Build history of the part. All positions in model axes, mm. A direction names the side the tool comes from. Coordinates: 2 decimals unless noted, no trailing zeros. Loops run counter-clockwise (first coordinate to the right, second up) from the corner with the lowest first, then second, coordinate; pieces in that order, holes last.
(1) Tool access for faces 1 (the face through (-151.49, 51.39, 24.45)), 2 (the face through (-77.27, 0.91, 24.45)), 3 (the face through (-75, 98.425, 5)), 4 (the face through (-75, 6.35, 19)), 5 (the face through (-0.91, 51.39, 24.45)): list every direction of +Z, -Z, +X, -X, +Y, -Y with a clear straight run to the whole face (end or side of a thin tool).
(2) Flat gauge pins, fed straight in: P1, Ø2.5, axis at x = -66.5, y = 5, coming from the +Z side; P2, Ø23, axis at x = -71.5, y = 43, coming from the -Z side (3 decimals); P3, Ø0.8, axis at x = -13.5, z = 26.5, coming from the +Y side. Where does each tip first touch, or does it go through?
(3) Slice it at B-B (x = -34.5). Give the cut face in (y, z) (3 decimals), and give its area (3 significant figures).
(4) Slice it at A-A (z = 4). Give the cut face in (x, y) (3 decimals), and give its area (3 significant figures).
(5) Wall check: L1, parallel to Y at x = -60, z = 16 (3 decimals); L2, parallel to X at y = 44, z = 14 (3 decimals); L3, parallel to X at y = 55.5, z = 26.75. Give the ranges that are in metal, low to high.
(6) Two-plate mould, pull along Y, no slides. Class faces 6 (the face through (-75, 5, 25.4)), 7 (the face through (-77.27, 100.69, 24.45)), 8 (the face through (-77, 94, 9.525)): pulls with the +Y half, pulls with the -Y half, needs draft (parallel to the pull), parting line crosses it, or undercut.
(7) Slice it at C-C (y = 21). Give the cut face in (x, z) (3 decimals).
from build123d import *

# Parameters (mm, degrees)
F0_W        = 101.6
F0_H        = 25.4
F1_DEPTH    = 152.4
F2_W        = 2.54
F2_H        = 12.7
F3_DEPTH    = 152.401
F4_W        = 1.524
F4_H        = 71.12
F5_DEPTH    = 2.54
F6_R        = 3.175
F7_T        = 3.175
F7_T3_DEPTH = 158.75
F7_T5_DEPTH = 77.47
F7_T7_DEPTH = 7.874
F7_T9_DEPTH = 7.874


# Not quite as in the source:
# - a shell that OpenCascade refuses in one call is made with other operations: the cavity is built on its own and cut out


with BuildPart() as f1:
    # F0 (on Right) → F1 (new body)
    with BuildSketch(Plane.YZ):
        with Locations((50.8, 12.7)):
            Rectangle(F0_W, F0_H)
    extrude(amount=-F1_DEPTH)

    # F2 (on face) → F3 (cut, through all)
    with BuildSketch(Plane.YZ):
        with Locations((7.62, 19.05)):
            Rectangle(F2_W, F2_H)
        with Locations((93.98, 19.05)):
            Rectangle(F2_W, F2_H)
    extrude(amount=-F3_DEPTH, mode=Mode.SUBTRACT)

    # F4 (on face) → F5 (join)
    with BuildSketch(Plane.XY.offset(25.4)):
        with Locations((-138.938, 50.8)):
            Rectangle(F4_W, F4_H)
        with Locations((-13.462, 50.8)):
            Rectangle(F4_W, F4_H)
    extrude(amount=F5_DEPTH)

    # F6
    f6_edges = [f1.edges().sort_by_distance(p)[0] for p in [
        (-76.2, 0, 25.4),
        (-76.2, 101.6, 25.4),
        (0, 50.8, 25.4),
        (-152.4, 50.8, 25.4),
    ]]
    fillet(f6_edges, radius=F6_R)

    # F7: shell of thickness 3.175, made by hand


with BuildPart() as f7_core1:
    # F7_t2: copy of F1
    add(f1.part)

    # the walls: a layer under each face that stays
    f7_faces = [f7_core1.faces().sort_by_distance(p)[0] for p in [
        (-76.2, 0, 11.1125),
        (0, 50.8, 12.7),
        (-152.4, 50.8, 12.7),
        (-76.2, 4.7625, 25.4),
        (-76.2, 6.35, 19.05),
        (-76.2, 7.62, 12.7),
        (-76.2, 8.89, 19.05),
        (-76.2, 101.6, 11.1125),
        (-76.2, 92.71, 19.05),
        (-76.2, 96.8375, 25.4),
        (-76.2, 93.98, 12.7),
        (-76.2, 95.25, 19.05),
        (-76.2, 50.8, 25.4),
        (-138.176, 50.8, 26.67),
        (-138.938, 86.36, 26.67),
        (-139.7, 50.8, 26.67),
        (-138.938, 15.24, 26.67),
        (-12.7, 50.8, 26.67),
        (-13.462, 86.36, 26.67),
        (-14.224, 50.8, 26.67),
        (-13.462, 15.24, 26.67),
        (-138.938, 50.8, 27.94),
        (-13.462, 50.8, 27.94),
    ]]
    thicken(f7_faces, amount=-F7_T, mode=Mode.SUBTRACT)

    # F7_s4 → F7_t3 (cut)
    with BuildSketch(Plane.YZ.offset(-155.575)):
        Polygon((6.38175, 12.73175), (3.175, 12.7), (3.175, 9.525), (6.35, 9.525), align=None)
        Polygon((8.85825, 12.73175), (8.89, 9.525), (12.065, 9.525), (12.065, 12.7), align=None)
        Polygon((92.74175, 12.73175), (89.535, 12.7), (89.535, 9.525), (92.71, 9.525), align=None)
        Polygon((95.21825, 12.73175), (95.25, 9.525), (98.425, 9.525), (98.425, 12.7), align=None)
    extrude(amount=F7_T3_DEPTH, mode=Mode.SUBTRACT)

    # F7_s6 → F7_t5 (cut)
    with BuildSketch(Plane.XZ.offset(-89.535)):
        Polygon((-138.14425, 25.43175), (-138.176, 22.225), (-141.351, 22.225), (-141.351, 25.4), align=None)
        Polygon((-139.73175, 25.43175), (-139.7, 22.225), (-136.525, 22.225), (-136.525, 25.4), align=None)
        Polygon((-12.66825, 25.43175), (-12.7, 22.225), (-15.875, 22.225), (-15.875, 25.4), align=None)
        Polygon((-14.25575, 25.43175), (-14.224, 22.225), (-11.049, 22.225), (-11.049, 25.4), align=None)
    extrude(amount=F7_T5_DEPTH, mode=Mode.SUBTRACT)

    # F7_s8 → F7_t7 (cut)
    with BuildSketch(Plane.YZ.offset(-142.875)):
        Polygon((86.39175, 25.43175), (86.36, 22.225), (83.185, 22.225), (83.185, 25.4), align=None)
        Polygon((15.20825, 25.43175), (15.24, 22.225), (18.415, 22.225), (18.415, 25.4), align=None)
    extrude(amount=F7_T7_DEPTH, mode=Mode.SUBTRACT)

    # F7_s10 → F7_t9 (cut)
    with BuildSketch(Plane.YZ.offset(-17.399)):
        Polygon((86.39175, 25.43175), (86.36, 22.225), (83.185, 22.225), (83.185, 25.4), align=None)
        Polygon((15.20825, 25.43175), (15.24, 22.225), (18.415, 22.225), (18.415, 25.4), align=None)
    extrude(amount=F7_T9_DEPTH, mode=Mode.SUBTRACT)


with BuildPart() as f1_1:
    add(f1.part)

    # what is left inside the walls is the cavity
    f7_cavity = [f7_core1.part.solids().sort_by_distance(p)[0] for p in [
        (-100.541667, 50.8, 0.03175),
    ]]
    add(f7_cavity, mode=Mode.SUBTRACT)


solid = f1_1.part
Response values:
1. face 1: +Z, -X
1. face 2: +Z, +X, -X, -Y
1. face 3: -Z
1. face 4: +Z, +X, -X
1. face 5: +Z, +X
2. P1: stops at z = 25.4
2. P2: stops at z = 22.225
2. P3: stops at y = 86.36
3. outline: (0, 0) - (3.175, 0) - (3.175, 9.525) - (12.065, 9.525) - (12.065, 22.225) - (89.535, 22.225) - (89.535, 9.525) - (98.425, 9.525) - (98.425, 0) - (101.6, 0) - (101.6, 22.225) arc R3.175 ccw to (98.425, 25.4) - (95.25, 25.4) - (95.25, 12.7) - (92.71, 12.7) - (92.71, 25.4) - (8.89, 25.4) - (8.89, 12.7) - (6.35, 12.7) - (6.35, 25.4) - (3.175, 25.4) arc R3.175 ccw to (0, 22.225) - close
3. area: 621 mm2
4. outline: (-152.4, 0) - (0, 0) - (0, 101.6) - (-152.4, 101.6) - close; hole (-149.225, 3.175) - (-3.175, 3.175) - (-3.175, 98.425) - (-149.225, 98.425) - close
4. area: 1,570 mm2
5. L1: y = 0 to 6.35, 8.89 to 12.065, 89.535 to 92.71, 95.25 to 101.6
5. L2: x = -152.4 to -149.225, -3.175 to 0
5. L3: x = -139.7 to -138.18, -14.22 to -12.7
6. face 6: needs draft
6. face 7: pulls with the +Y half
6. face 8: undercut
7. outline: (-152.4, 0) - (-149.225, 0) - (-149.225, 22.225) - (-3.175, 22.225) - (-3.175, 0) - (0, 0) - (0, 22.225) arc R3.175 ccw to (-3.175, 25.4) - (-12.7, 25.4) - (-12.7, 27.94) - (-14.224, 27.94) - (-14.224, 25.4) - (-138.176, 25.4) - (-138.176, 27.94) - (-139.7, 27.94) - (-139.7, 25.4) - (-149.225, 25.4) arc R3.175 ccw to (-152.4, 22.225) - close
